Work out the finished part from the listing and answer in its coordinate system (mm). Round coordinates to 2 decimals unless told otherwise and drop trailing zeros. Write each loop counter-clockwise with the first axis right and the second up, starting at its lowest first coordinate (ties: lowest second). Pieces come first, ordered by that corner, then holes. Notation, with made-up numbers: (51, 28.25) -> (94, 28.25) arc R16 ccw to (94, 47.25) -> close; hole circle Ø11 at (-28.75, 70.25). An arc over 180 degrees is marked (long way). One line per item, written item: value.
```python
from build123d import *

# Parameters (mm, degrees)
SKETCH1_R           = 1.5
BOSS_EXTRUDE1_DEPTH = 1.5
FILLET1_R           = 20
FILLET2_R           = 20


with BuildPart() as part:
    # Sketch1 → Boss-Extrude1 (new body)
    with BuildSketch(Plane.XY):
        with BuildLine():
            Line((-4.311554675, 0), (20.688445325, 0))
            add(Edge.make_bspline(
                [(20.688445325, 0), (60.31282649, -111.601969695), (18.819240624, -205)],
                knots=[0, 0, 0, 0.94797239, 0.94797239, 0.94797239], degree=2))
            Line((18.819240624, -205), (-146.979240624, -205))
            add(Edge.make_bspline(
                [(-148.848445325, 0), (-188.47282649, -111.601969695), (-146.979240624, -205)],
                knots=[0, 0, 0, 0.94797239, 0.94797239, 0.94797239], degree=2))
            Line((-148.848445325, 0), (-123.848445325, 0))
            add(Edge.make_bspline(
                [(-123.848445325, 0), (-138.20220228, -108.592832155), (-123.848445325, -180)],
                knots=[0, 0, 0, 0.806546207, 0.806546207, 0.806546207], degree=2))
            Line((-123.848445325, -180), (-4.311554675, -180))
            add(Edge.make_bspline(
                [(-4.311554675, 0), (10.04220228, -108.592832155), (-4.311554675, -180)],
                knots=[0, 0, 0, 0.806546207, 0.806546207, 0.806546207], degree=2))
        make_face()
        with Locations((2.285, -10)):
            Circle(SKETCH1_R, mode=Mode.SUBTRACT)
        with Locations((15.025, -10)):
            Circle(SKETCH1_R, mode=Mode.SUBTRACT)
        with Locations(Location((-143.185, -10, 0), (0, 0, 180))):
            Circle(SKETCH1_R, mode=Mode.SUBTRACT)
        with Locations(Location((-130.445, -10, 0), (0, 0, 180))):
            Circle(SKETCH1_R, mode=Mode.SUBTRACT)
    extrude(amount=BOSS_EXTRUDE1_DEPTH)

    # Fillet1
    fillet1_edges = [part.edges().sort_by_distance(p)[0] for p in [
        (-123.848445325, -180, 0.75),
        (-4.311554675, -180, 0.75),
    ]]
    fillet(fillet1_edges, radius=FILLET1_R)

    # Fillet2
    fillet2_edges = [part.edges().sort_by_distance(p)[0] for p in [
        (-146.979240624, -205, 0.75),
        (18.819240624, -205, 0.75),
    ]]
    fillet(fillet2_edges, radius=FILLET2_R)


solid = part.part
```
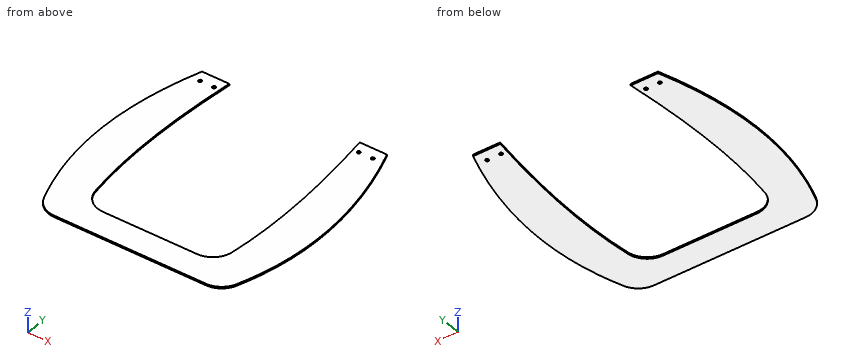
(1) Find section B-B on x = -98. Give the vertices of the cut face in (y, z), plus the area to 3 significant figures.
Reported:
outline: (-205, 0) -> (-180, 0) -> (-180, 1.5) -> (-205, 1.5) -> close
area: 37.5 mm2
(2) Consider probe 1 along X at (y, z) = (-153, 0.55); probe 2 along Y at (x, z) = (-27, 0.75); probe 3 along X at (y, z) = (-38, 0.9). Determine where each line is inside the solid, lowest interval first.
Reported:
probe 1: x = -163.52 to -128.1, -0.06 to 35.36
probe 2: y = -205 to -180
probe 3: x = -160.11 to -128.1, -0.06 to 31.95
(3) Flat-ended cylindrical pins translate along their axes: pin 1 Ø1.8 at (x, y) = (-143.185, -10) entering from -Z; pin 2 Ø0.8 at (x, z) = (-74.5, 1) entering from +Y. Find the tip coordinate at first contact, or state that the pin passes through.
Reported:
pin 1: passes through
pin 2: stops at y = -180
(4) Find section A-A on z = 0.8. Give the number of separate pieces and of enclosed holes in the cut face, plus the area to 3 significant figures.
Reported:
separate pieces: 1
enclosed holes: 4
area: 16,700 mm2
